Input: part model. Units: mm. Frame: model coordinates. Face numbers are marked on the shaded views. Round coordinates to 2 decimals unless told otherwise and drop trailing zeros. Loops run counter-clockwise (first coordinate to the right, second up) from the corner with the lowest first, then second, coordinate; pieces in that order, holes last. Notation, with made-up numbers: (-38.75, 32) -> (-29.75, 32) arc R16 ccw to (-29.75, 41) -> close; hole circle Ø2 at (53, 22). An arc over 180 degrees is marked (long way). Answer as a JSON object with one key per item and string values. Group by question number.
Item 1: Pin query (flat end, axial travel): pin 1 (5 mm diameter, centred on x = 9.5, z = -1, fed in from -Y). Return the tip coordinate at first contact, or that it passes through.
Item 2: Section query B-B on x = -7. Return loops of the section in (y, z).
Item 3: Section query C-C on x = 7. Return loops of the section in (y, z), and give its area (3 significant figures).
Item 4: Draft query along X for the marked faces 1, 2 and 3. Return one class per face: released by +X, released by -X, zero draft, split by the parting line, or undercut.
Item 5: Material intervals for line 1 (Y direction, x = 6, z = 7.25); line 2 (X direction, y = 14, z = -7); line 3 (Z direction, x = -11.75, y = 20.5), sorted ascending. Write a range as [from, to].
Item 6: Section query A-A on z = 0. Return loops of the section in (x, y), and give its area (3 significant figures).
Item 7: Section query D-D on z = -5.75. Return loops of the section in (x, y), and give its area (3 significant figures).
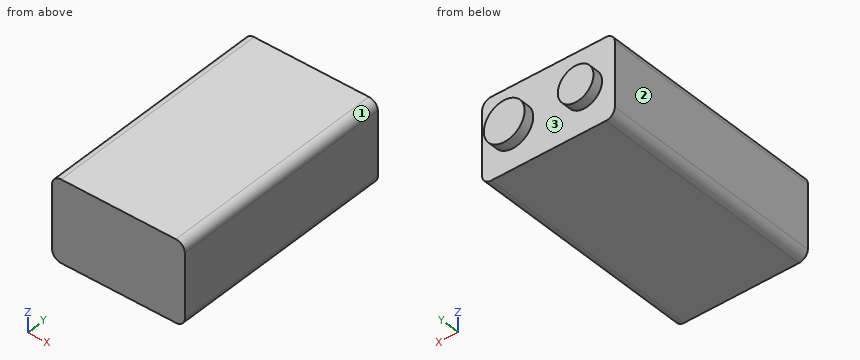
from build123d import *

# Parameters (mm, degrees)
SKETCH1_W           = 26
SKETCH1_H           = 16
BOSS_EXTRUDE1_DEPTH = 45
SKETCH2_R           = 3.5
SKETCH2_R_2         = 4
BOSS_EXTRUDE2_DEPTH = 2
FILLET1_R           = 1.75


with BuildPart() as part:
    # Sketch1 → Boss-Extrude1 (new body)
    with BuildSketch(Plane(origin=(0, 0, 0), x_dir=(1, 0, 0), z_dir=(0, 1, 0))):
        Rectangle(SKETCH1_W, SKETCH1_H)
    extrude(amount=BOSS_EXTRUDE1_DEPTH)

    # Sketch2 → Boss-Extrude2 (add)
    with BuildSketch(Plane(origin=(0, 45, 0), x_dir=(1, 0, 0), z_dir=(0, 1, 0))):
        with Locations((-7, 0)):
            Circle(SKETCH2_R)
        with Locations((7, 0)):
            Circle(SKETCH2_R_2)
    extrude(amount=BOSS_EXTRUDE2_DEPTH)

    # Fillet1
    fillet1_edges = [part.edges().sort_by_distance(p)[0] for p in [
        (13, 22.5, 8),
        (-13, 22.5, 8),
        (-13, 22.5, -8),
        (13, 22.5, -8),
    ]]
    fillet(fillet1_edges, radius=FILLET1_R)


solid = part.part
Solved:
{
 "1": {"pin 1": "y = 0"},
 "2": {"outline": "(0, -8) -> (45, -8) -> (45, -3.5) -> (47, -3.5) -> (47, 3.5) -> (45, 3.5) -> (45, 8) -> (0, 8) -> close"},
 "3": {"outline": "(0, -8) -> (45, -8) -> (45, -4) -> (47, -4) -> (47, 4) -> (45, 4) -> (45, 8) -> (0, 8) -> close", "area": "736 mm²"},
 "4": {"face 1": "released by +X", "face 2": "released by -X", "face 3": "undercut"},
 "5": {"line 1": "[0, 45]", "line 2": "[-12.83, 12.83]", "line 3": "[-7.93, 7.93]"},
 "6": {"outline": "(-13, 0) -> (13, 0) -> (13, 45) -> (11, 45) -> (11, 47) -> (3, 47) -> (3, 45) -> (-3.5, 45) -> (-3.5, 47) -> (-10.5, 47) -> (-10.5, 45) -> (-13, 45) -> close", "area": "1,200 mm²"},
 "7": {"outline": "(-13, 0) -> (13, 0) -> (13, 45) -> (-13, 45) -> close", "area": "1,170 mm²"}
}
